```python
from build123d import *

# Parameters (mm, degrees)
F0_R      = 6
F1_DEPTH  = 3
F2_R      = 5.75
F3_DEPTH  = 1.15
F4_R      = 6
F4_R_2    = 5.75
F5_DEPTH  = 16
F6_R      = 8
F6_R_2    = 6
F7_DEPTH  = 872
F8_R      = 6
F9_DEPTH  = 15
F10_R     = 5.95
F11_DEPTH = 2
F12_R     = 5.95
F13_DEPTH = 3
F14_R     = 5
F15_DEPTH = 15
F16_SIZE  = 1


with BuildPart() as f1:
    # F0 (on Top) → F1 (new body)
    with BuildSketch(Plane.XY):
        Circle(F0_R)
    extrude(amount=F1_DEPTH)

    # F2 (on face) → F3 (join)
    with BuildSketch(Plane.XY.offset(3)):
        Circle(F2_R)
    extrude(amount=F3_DEPTH)

    # F4 (on face) → F5 (join)
    with BuildSketch(Plane.XY.offset(4.15)):
        Circle(F4_R)
        Circle(F4_R_2, mode=Mode.SUBTRACT)
        Circle(F4_R_2)
    extrude(amount=F5_DEPTH)

    # F6 (on face) → F7 (join)
    with BuildSketch(Plane.XY.offset(20.15)):
        Circle(F6_R)
        Circle(F6_R_2, mode=Mode.SUBTRACT)
        Circle(F6_R_2)
    extrude(amount=F7_DEPTH)

    # F8 (on face) → F9 (join)
    with BuildSketch(Plane.XY.offset(892.15)):
        Circle(F8_R)
    extrude(amount=F9_DEPTH)

    # F10 (on face) → F11 (join)
    with BuildSketch(Plane.XY.offset(907.15)):
        Circle(F10_R)
    extrude(amount=F11_DEPTH)

    # F12 (on face) → F13 (join)
    with BuildSketch(Plane.XY.offset(909.15)):
        Circle(F12_R)
    extrude(amount=F13_DEPTH)

    # F14 (on face) → F15 (join)
    with BuildSketch(Plane.XY.offset(912.15)):
        Circle(F14_R)
    extrude(amount=F15_DEPTH)

    # F16
    f16_edges = [f1.edges().sort_by_distance(p)[0] for p in [
        (-5, 0, 927.15),
        (-6, 0, 0),
    ]]
    chamfer(f16_edges, length=F16_SIZE)


solid = f1.part
```
Input: part model. Units: mm. Frame: model coordinates. A direction names the side the tool comes from. Give positions to 0.01 mm unless a question says otherwise; leave off trailing zeros. Write each loop counter-clockwise with the first axis right and the second up, starting at its lowest first coordinate (ties: lowest second). Pieces come first, ordered by that corner, then holes. Notation, with made-up numbers: (76, 36.25) - (114, 36.25) arc R17 cw to (114, 55.25) - close; hole circle Ø4 at (0.5, -17.5). An arc over 180 degrees is marked (long way). Write item = value, one per line. Start each with the question number.
1) Material intervals for L1, parallel to Z at x = 6.5, y = -1; L2, parallel to X at y = 0.75, z = 99.5; L3, parallel to X at y = 5.25, z = 349, sorted ascending. Write a range as [from, to].
2) Pin query (flat end, axial travel): pin 1 (5 mm diameter, centred on x = -4, z = 466, fed in from +Y); pin 2 (6 mm diameter, centred on y = -4.5, z = 533.5, fed in from -X); pin 3 (2 mm diameter, centred on x = 5.5, y = 4, fed in from -Z). Return the tip coordinate at first contact, or that it passes through.
3) Reachability of faces 1 (the face through (-2, 6, 892.15)), 2 (the face through (-2, 6, 20.15)), 3 (the face through (-1.73, -7.81, 450.05)) from +Z, -Z, +X, -X, +Y, -Y: full face, straight path, thin tool, end or side. Return the list, or none.
4) Cut plane C-C (z = 281). Return loops of the section in (x, y), and give its area (3 significant figures).
Answers follow:
q1.L1 = [20.15, 892.15]
q1.L2 = [-7.96, 7.96]
q1.L3 = [-6.04, 6.04]
q2.pin_1 = 7.86
q2.pin_2 = -7.86
q2.pin_3 = 0.8
q3.face_1 = +Z
q3.face_2 = -Z
q3.face_3 = +Z, -Z
q4.outline = circle Ø16 at (0, 0)
q4.area = 201 mm^2
